from build123d import *

# Parameters (mm, degrees)
F1_DEPTH = 304.8
F3_D     = 12.7
F4_W     = 27.686
F4_H     = 215.9
F4_H_2   = 254
F5_DEPTH = 27.94
F6_W     = 23.114
F6_H     = 520.7
F7_DEPTH = 10.161


# Not quite as in the source:
# - a length typed as a fraction of an inch, garbled in the dataset ("3 / 203.2 mm" for 3/8 in), is restored


with BuildPart() as f1:
    # F0 (on Front) → F1 (new body, symmetric)
    with BuildSketch(Plane.XZ):
        Polygon((0, 27.94), (0, 0), (27.686, 0), (27.686, 38.1), (-23.114, 38.1), (-23.114, 27.94), align=None)
    extrude(amount=F1_DEPTH, both=True)

    # F3 (through all)
    with Locations(Plane(origin=(0, 0, 0), x_dir=(1, 0, 0), z_dir=(0, 0, -1))):
        with Locations((12.7, 25.4), (12.7, -279.4)):
            Hole(F3_D / 2)

    # F4 (on face) → F5 (cut, through all)
    with BuildSketch(Plane(origin=(0, 0, 0), x_dir=(1, 0, 0), z_dir=(0, 0, -1))):
        with Locations((13.843, 196.85)):
            Rectangle(F4_W, F4_H)
        with Locations((13.843, -127)):
            Rectangle(F4_W, F4_H_2)
    extrude(amount=-F5_DEPTH, mode=Mode.SUBTRACT)

    # F6 (on face) → F7 (cut, through all)
    with BuildSketch(Plane(origin=(0, 0, 27.94), x_dir=(1, 0, 0), z_dir=(0, 0, -1))):
        with Locations((-11.557, -44.45)):
            Rectangle(F6_W, F6_H)
    extrude(amount=-F7_DEPTH, mode=Mode.SUBTRACT)


solid = f1.part
Check sheet for the modelled part. Datum: model origin and axes. Units: mm. A direction names the side the tool comes from. Give positions to 0.01 mm unless a question says otherwise; leave off trailing zeros. Write each loop counter-clockwise with the first axis right and the second up, starting at its lowest first coordinate (ties: lowest second). Pieces come first, ordered by that corner, then holes. Notation, with made-up numbers: (87, -29) -> (93, -29) arc R12 cw to (93, -24) -> close; hole circle Ø2 at (49, 72.25). An arc over 180 degrees is marked (long way). One line per item, written item: value. Start each with the question number.
Item 1: Section check B-B on y = 279.4. Record the cut outline in (x, z).
Item 2: Material ranges on probe 1 along Y at (x, z) = (12.7, 11); probe 2 along Y at (x, z) = (12.7, 30.5); probe 3 along X at (y, z) = (279, 30), recorded low to high. Write a range as from..to.
Item 3: Draft check along Y on faces 1 (the cylindrical face through (13.5, 273.1, 19.3)), 2 (the flat face through (14, -88.9, 14)), 3 (the flat face through (20, 279, 0)). Enter one of: +Y half, -Y half, draft (parallel to the pull), parting line (faces both ways), or undercut.
Item 4: Gauge pin test, flat ends, axial feed: pin 1 (12 mm diameter, centred on y = -32.5, z = 32, fed in from -X); pin 2 (12 mm diameter, centred on x = 15, y = 100, fed in from -Z); pin 3 (3 mm diameter, centred on x = 11.5, z = 13, fed in from -Y). Record the tip position at first contact, or that the pin passes through.
Item 5: Section check A-A on z = 14.5. Record the cut outline in (x, y), then the cut area to 3 significant figures.
Item 6: Tool access check on faces 4 (the flat face through (2, -304.8, 33)), 5 (the flat face through (8, -222, 27.94)), 6 (the flat face through (-23.114, -261, 33)), 7 (the flat face through (-12, -215.9, 33)), 8 (the flat face through (14, 125, 27.94)). Record the directions out of +Z, -Z, +X, -X, +Y, -Y that give a thin tool (end or side, any length) a straight path to the whole face; none if there is none.
Item 7: Section check C-C on x = 12.7. Record the cut outline in (y, z).
Item 8: Section check D-D on x = -9. Record the cut outline in (y, z).
Results list:
1. outline: (0, 0) -> (6.35, 0) -> (6.35, 38.1) -> (0, 38.1) -> close; (19.05, 0) -> (27.69, 0) -> (27.69, 38.1) -> (19.05, 38.1) -> close
2. probe 1: -88.9..-31.75, -19.05..0, 254..273.05, 285.75..304.8
2. probe 2: -304.8..-31.75, -19.05..273.05, 285.75..304.8
2. probe 3: 0..6.36, 19.04..27.69
3. face 1: undercut
3. face 2: -Y half
3. face 3: draft
4. pin 1: x = 0
4. pin 2: z = 27.94
4. pin 3: y = -88.9
5. outline: (0, -88.9) -> (27.69, -88.9) -> (27.69, 0) -> (0, 0) -> close; (0, 254) -> (27.69, 254) -> (27.69, 304.8) -> (0, 304.8) -> close; hole circle Ø12.7 at (12.7, -25.4); hole circle Ø12.7 at (12.7, 279.4)
5. area: 3,610 mm²
6. face 4: +Z, -Z, +X, -X, -Y
6. face 5: -Z, +X, -X, -Y
6. face 6: +Z, -Z, -X, +Y, -Y
6. face 7: +Z, -Z, -X, +Y
6. face 8: -Z, +X, -X
7. outline: (-304.8, 27.94) -> (-88.9, 27.94) -> (-88.9, 0) -> (-31.75, 0) -> (-31.75, 38.1) -> (-304.8, 38.1) -> close; (-19.05, 0) -> (0, 0) -> (0, 27.94) -> (254, 27.94) -> (254, 0) -> (273.05, 0) -> (273.05, 38.1) -> (-19.05, 38.1) -> close; (285.75, 0) -> (304.8, 0) -> (304.8, 38.1) -> (285.75, 38.1) -> close
8. outline: (-304.8, 27.94) -> (-215.9, 27.94) -> (-215.9, 38.1) -> (-304.8, 38.1) -> close
